Autodesk Fusion 360 part; units mm, degrees
sketch "Sketch1" plane through (0, 0, 0) normal (0, 0, 1) x (1, 0, 0)
  line L0 (5, 1.75) -> (-5, 1.75)
  line L1 (-5, 1.75) -> (-5, -1.75)
  line L2 (-5, -1.75) -> (5, -1.75)
  line L3 (5, -1.75) -> (5, 1.75)
  line L4 (5, 1.75) -> (-5, -1.75) construction
  line L5 (-5, 1.75) -> (5, -1.75) construction
  line L6 (-7, -3.75) -> (7, -3.75)
  line L7 (7, -3.75) -> (7, 3.75)
  line L8 (7, 3.75) -> (-7, 3.75)
  line L9 (-7, 3.75) -> (-7, -3.75)
  dimension "d1" = 10
  dimension "d2" = 3.5
  dimension "d3" = 2
extrude "Extrude1" add sketch "Sketch1" along normal blind 6
fillet "Fillet2" radius 1.5 4 edges at (7, 3.75, 3) (-7, 3.75, 3) (-7, -3.75, 3) (7, -3.75, 3)
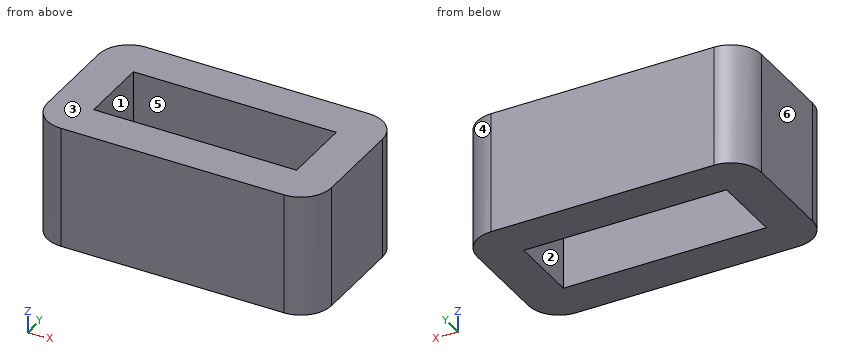
Source: CAD feature listing. Evaluate the final solid. Frame: model axes, mm. Face numbers are marked on the shaded views. A direction names the side the tool comes from. Round coordinates to 2 decimals unless told otherwise and drop trailing zeros. Loops run counter-clockwise (first coordinate to the right, second up) from the corner with the lowest first, then second, coordinate; pieces in that order, holes last. Notation, with made-up numbers: M -11,-31 L 33,-31 A22 cw 33,-22 Z; hole C 43.5,9 d11. An arc over 180 degrees is marked long. Put each result on its own line as item: value.
(1) Section D-D, the plane y = 3.25. Return loops of the section in (x, z), and give its area (3 significant figures).
Solutions:
outline: M -6.62,0 L 6.62,0 L 6.62,6 L -6.62,6 Z
area: 79.4 mm²
(2) Ray query, line 1 (Y direction, x = 0.75, z = 0.2); line 2 (X direction, y = 1.25, z = 1.95); line 3 (Y direction, x = 6.5, z = 3.95). Return the intervals inside material, ascending. Write a range as [from, to].
Solutions:
line 1: [-3.75, -1.75], [1.75, 3.75]
line 2: [-7, -5], [5, 7]
line 3: [-3.37, 3.37]
(3) Section B-B, the plane y = 0.25. Return loops of the section in (x, z).
Solutions:
outline: M -7,0 L -5,0 L -5,6 L -7,6 Z; M 5,0 L 7,0 L 7,6 L 5,6 Z
(4) Section C-C, the plane z = 3.25. Return loops of the section in (x, y), and give its area (3 significant figures).
Solutions:
outline: M -7,-2.25 A1.5 ccw -5.5,-3.75 L 5.5,-3.75 A1.5 ccw 7,-2.25 L 7,2.25 A1.5 ccw 5.5,3.75 L -5.5,3.75 A1.5 ccw -7,2.25 Z; hole M -5,-1.75 L 5,-1.75 L 5,1.75 L -5,1.75 Z
area: 68.1 mm²
(5) Access query for the marked faces 5 and 6. Directions: +Z, -Z, +X, -X, +Y, -Y. A direction counts if a zero-diameter tool reaches every point of the face in a straight line with its end or side. Return the directions, or none.
Solutions:
face 5: +Z, -Z
face 6: +Z, -Z, -X, +Y, -Y
(6) Section A-A, the plane x = 1. Return loops of the section in (y, z).
Solutions:
outline: M -3.75,0 L -1.75,0 L -1.75,6 L -3.75,6 Z; M 1.75,0 L 3.75,0 L 3.75,6 L 1.75,6 Z
(7) First-contact query: pin 1 (1.5 mm diameter, centred on x = -3, y = 0.5, fed in from +Z). Flat tip, straight axial feed; report the tip coordinate or a pass-through.
Solutions:
pin 1: through
(8) Pull-direction query (X, two-part tool) for the marked faces 1, 2, 3 and 4; classes: released by +X, released by -X, zero draft, split by the parting line, or undercut.
Solutions:
face 1: undercut
face 2: undercut
face 3: zero draft
face 4: released by +X
